Here's how the part is built. I have some questions about the finished solid (model axes, mm). A direction names the side the tool comes from. Give positions to 0.01 mm unless a question says otherwise; leave off trailing zeros. Order: outer loops, then holes, each group sorted by start corner. A loop starts at its lowest first (then second) coordinate and runs counter-clockwise, first axis right, second up. Notation, with made-up numbers: (4.25, -8.5) -> (59.25, -8.5) arc R21 ccw to (59.25, 28.5) -> close; hole circle Ø8 at (31.5, -15.75). An arc over 180 degrees is marked (long way). Write each question's results on one line, items separated by ' | '. Start each with the question number.
Q1. Imagine slicing it at A-A, the plane z = 23. Please give me the cut outline in (x, y).
Q2. I'm going to push flat-ended pins straight in: pin 1 (6 mm diameter, centred on x = 40.5, z = 3, fed in from +Y); pin 2 (3 mm diameter, centred on x = 16.5, z = 12.5, fed in from -Y); pin 3 (4.5 mm diameter, centred on x = 0, z = 0, fed in from -Y). Where does each tip first touch, or does it pass through?
Q3. Imagine slicing it at B-B, the plane z = 43. Please give me the cut outline in (x, y).
Q4. Imagine slicing it at C-C, the plane x = 29.5. Please give me the cut outline in (y, z), then the cut area to 3 significant figures.
Q5. I need wall thicknesses on line 1 along Z through (x, y) = (30.5, 9.5); line 2 along Z through (x, y) = (45.5, 2.25); line 3 along X through (y, z) = (6, -16.5). Which ranges of each line are inside material? Lowest first, please. Write a range as [from, to].
Q6. For faces 4 (the face through (6, 5, -8)), 5 (the face through (-20.225, 4.977, 60.196)), which set-ups out of +Z, -Z, +X, -X, +Y, -Y let a thin tool reach every point of the face, with its end or its side?
Q7. Thinking about a two-plate mould opening in Z: for faces 1 (the face through (8.98, 4.93, 34.61)), 2 (the face through (29.67, 5.07, 20.41)), 3 (the face through (5, 0, 0)), which applies, pulls with the +Z half, pulls with the -Z half, needs draft (parallel to the pull), parting line crosses it, or undercut?
Autodesk Inventor part; units mm, degrees
ref_plane "YZ Plane" through (0, 0, 0) normal (1, 0, 0) x (0, 1, 0)
ref_plane "XZ Plane" through (0, 0, 0) normal (0, 1, 0) x (-1, 0, 0)
ref_plane "XY Plane" through (0, 0, 0) normal (0, 0, 1) x (1, 0, 0)
sketch "Sketch1" plane through (0, 0, 0) normal (0, 1, 0) x (-1, 0, 0)
  circle A0 centre (0, 0) radius 10
  dimension "d0" = 20
extrude "Extrusion1" add sketch "Sketch1" along normal blind 10
sketch "Sketch3" plane through (0, 0, 0) normal (1, 0, 0) x (0, 1, 0)
  line L0 (0, 5) -> (10, -0.7735)
  line L1 (10, -0.7735) -> (10, -3.7735)
  line L2 (10, -3.7735) -> (0, 2)
  line L3 (0, 2) -> (0, 5)
  point P0 (0, 0)
  dimension "d3" = 3
  dimension "d4" = 10
  dimension "d5" = 10
  dimension "d6" = 60
  dimension "d7" = 5
extrude "Extrusion2" add sketch "Sketch3" along normal blind 63.5
pattern_circular "Circular Pattern1" count 10 over 360 about axis through (0, 0, 0) along (0, 1, 0) of "Extrusion2"
sketch "Sketch4" plane through (0, 10, 0) normal (0, 1, 0) x (1, 0, 0)
  circle A0 centre (0, 0) radius 5
  dimension "d13" = 10
extrude "Extrusion3" add sketch "Sketch4" along normal blind 5
fillet "Fillet1" radius 5 1 edges at (-5, 15, 0)
sketch "Sketch5" plane through (0, 0, 0) normal (0, -1, 0) x (1, 0, 0)
  circle A0 centre (0, 0) radius 2.5
  dimension "d17" = 5
extrude "Extrusion4" cut sketch "Sketch5" against normal blind 2
properties part number "AERO - Propeller" material "ABS Plastic"
Geometry check:
1) outline: (-40.16, 0) -> (-35.06, 0) -> (-25.24, 10) -> (-30.34, 10) -> close; (-12.73, 0) -> (-9.58, 0) -> (-3.51, 10) -> (-6.66, 10) -> close; (2.22, 0) -> (5.37, 0) -> (11.44, 10) -> (8.29, 10) -> close; (23.15, 0) -> (28.25, 0) -> (38.08, 10) -> (32.97, 10) -> close
2) pin 1: y = 8.66 | pin 2: y = 0.15 | pin 3: y = 2
3) outline: (-19.23, 0) -> (-16.07, 0) -> (-10, 10) -> (-13.16, 10) -> close; (8.71, 0) -> (11.87, 0) -> (17.94, 10) -> (14.78, 10) -> close
4) outline: (0, -18.96) -> (10, -26.1) -> (10, -22.39) -> (0, -15.25) -> close; (0, 2) -> (10, -3.77) -> (10, -0.77) -> (0, 5) -> close; (0, 23.91) -> (10, 16.77) -> (10, 20.48) -> (0, 27.61) -> close | area: 104 mm²
5) line 1: [-26.47, -22.76], [-3.48, -0.48], [17.85, 21.56] | line 2: [-32.19, -28.48], [0.7, 3.7], [33.92, 37.63] | line 3: [-25.2, -20.1], [-6.9, -3.75], [3.82, 6.98], [20.22, 25.32]
6) face 4: none | face 5: +Z, -X, +Y, -Y
7) face 1: pulls with the +Z half | face 2: undercut | face 3: needs draft
